Model file for the job. Use its own axes, mm. Face numbers are marked on the shaded views. A direction names the side the tool comes from. Give positions to 0.01 mm unless a question says otherwise; leave off trailing zeros. Write each loop counter-clockwise with the first axis right and the second up, starting at its lowest first coordinate (ties: lowest second). Pieces come first, ordered by that corner, then holes. Notation, with made-up numbers: (-15, 27) - (-3, 27) arc R22 cw to (-3, 57) - close; hole circle Ø5 at (24, -3.5). An arc over 180 degrees is marked (long way). Use a Markdown table: item, result. Add a question column.
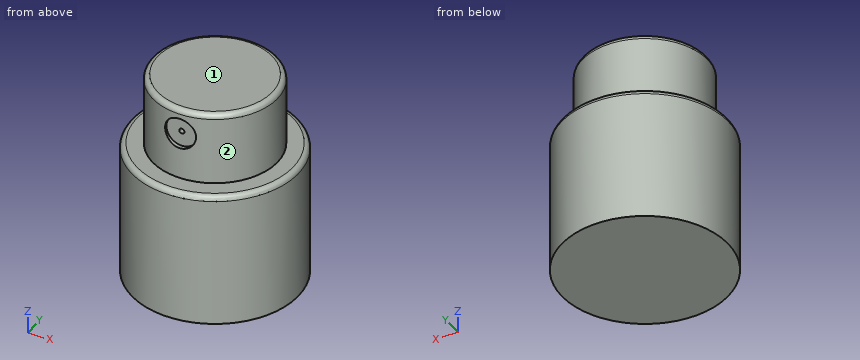
```python
from build123d import *

# Parameters (mm, degrees)
F0_R     = 6
F1_DEPTH = 20
F0_R_2   = 8
F2_DEPTH = 13
F4_R     = 0.25
F5_DEPTH = 23.7
F4_R_2   = 1.5
F6_DEPTH = 19.4
F7_R     = 0.5


with BuildPart() as f1:
    # F0 (on Top) → F1 (new body)
    with BuildSketch(Plane.XY):
        Circle(F0_R)
    extrude(amount=F1_DEPTH)

    # F0 (on Top) → F2 (join)
    with BuildSketch(Plane.XY):
        Circle(F0_R_2)
        Circle(F0_R, mode=Mode.SUBTRACT)
    extrude(amount=F2_DEPTH)

    # F4 (on offset) → F5 (cut)
    with BuildSketch(Plane.XZ.offset(25)):
        with Locations((0, 17.539654)):
            Circle(F4_R)
    extrude(amount=-F5_DEPTH, mode=Mode.SUBTRACT)

    # F4 (on offset) → F6 (cut)
    with BuildSketch(Plane.XZ.offset(25)):
        with Locations((0, 17.539654)):
            Circle(F4_R_2)
        with Locations((0, 17.539654)):
            Circle(F4_R, mode=Mode.SUBTRACT)
    extrude(amount=-F6_DEPTH, mode=Mode.SUBTRACT)

    # F7
    f7_edges = [f1.edges().sort_by_distance(p)[0] for p in [
        (-8, 0, 13),
        (-6, 0, 20),
    ]]
    fillet(f7_edges, radius=F7_R)


solid = f1.part
```
(1) Probe probe 1 along Z at (x, y) = (0, -4.4); probe 2 along Z at (x, y) = (0, -5.8); probe 3 along Y at (x, z) = (0, 16.5). List the from-to ranges inside material, lowest first. Write a range as [from, to].
(2) Which spindle directions (+Z, -Z, +X, -X, +Y, -Y) get a long thin tool onto all of the face, cutting with end or side? Do the marked faces 1 and 2. Say none if no direction does.
(3) Band-saw the part on C-C (z = 3.75). Write the cut outline in (x, y), then the cut area to 3 significant figures.
(4) Band-saw the part on D-D (z = 13.75). Write the cut outline in (x, y), then the cut area to 3 significant figures.
(5) Flat gauge pins, fed straight in: pin 1 (3.5 mm diameter, centred on x = 0, z = 17.54, fed in from +Y); pin 2 (1.5 mm diameter, centred on y = 2, z = 16, fed in from +X); pin 3 (1 mm diameter, centred on x = 5.5, z = 13, fed in from +Y); pin 4 (3 mm diameter, centred on y = 0.5, z = 10.5, fed in from +X). Where does each tip first touch, or does it go through?
(6) Band-saw the part on A-A (x = 0). Write the cut outline in (y, z), then the cut area to 3 significant figures.
(7) Band-saw the part on B-B (y = 0). Write the cut outline in (x, z).
Model answer:
| question | item | result |
|---|---|---|
| 1 | probe 1 | z = [0, 17.29], [17.79, 20] |
| 1 | probe 2 | z = [0, 16.04], [19.04, 19.9] |
| 1 | probe 3 | y = [-5.6, 6] |
| 2 | face 1 | +Z, +X, -X, +Y, -Y |
| 2 | face 2 | +Z |
| 3 | outline | circle Ø16 at (0, 0) |
| 3 | area | 201 mm^2 |
| 4 | outline | circle Ø12 at (0, 0) |
| 4 | area | 113 mm^2 |
| 5 | pin 1 | stops at y = 6 |
| 5 | pin 2 | stops at x = 5.87 |
| 5 | pin 3 | stops at y = 6.11 |
| 5 | pin 4 | stops at x = 8 |
| 6 | outline | (-8, 0) - (8, 0) - (8, 12.5) arc R0.5 ccw to (7.5, 13) - (6, 13) - (6, 19.5) arc R0.5 ccw to (5.5, 20) - (-5.5, 20) arc R0.5 ccw to (-6, 19.5) - (-6, 19.04) - (-5.6, 19.04) - (-5.6, 17.79) - (-1.3, 17.79) - (-1.3, 17.29) - (-5.6, 17.29) - (-5.6, 16.04) - (-6, 16.04) - (-6, 13) - (-7.5, 13) arc R0.5 ccw to (-8, 12.5) - close |
| 6 | area | 288 mm^2 |
| 7 | outline | (-8, 0) - (8, 0) - (8, 12.5) arc R0.5 ccw to (7.5, 13) - (6, 13) - (6, 19.5) arc R0.5 ccw to (5.5, 20) - (-5.5, 20) arc R0.5 ccw to (-6, 19.5) - (-6, 13) - (-7.5, 13) arc R0.5 ccw to (-8, 12.5) - close |
